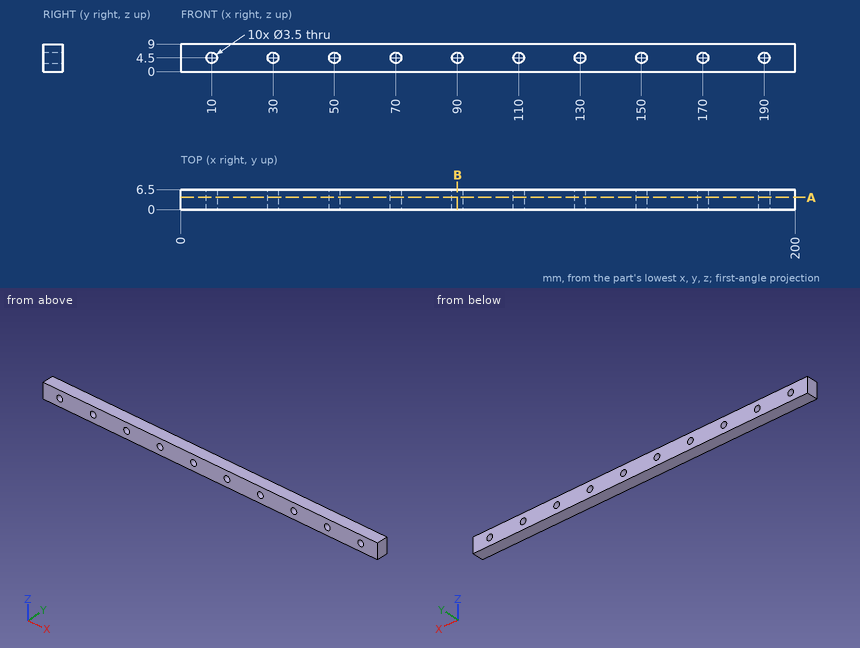
Print and shaded views of the part. All mm, measured from the part's lowest x, y and z. Round coordinates to 2 decimals unless told otherwise and drop trailing zeros. Write each loop counter-clockwise with the first axis right and the second up, starting at its lowest first coordinate (ties: lowest second). Pieces come first, ordered by that corner, then holes. Notation, with made-up numbers: (12, 20.25) -> (50, 20.25) arc R14 cw to (50, 28.25) -> close; hole circle Ø10 at (-9.75, -38.5). An arc over 180 degrees is marked (long way). Answer in a Markdown table with one row per item. Add a question column.
Item 1: Saw through at A-A, the plane y = 4. Count the separate pieces of the cut face and the enclosed holes in it, then the cut area to 3 significant figures.
Item 2: Saw through at B-B, the plane x = 90. Write the cut outline in (y, z), then the cut area to 4 significant figures.
Item 3: Drill centre line: line 1 (Z direction, x = 30, y = 1.5). Where is it in solid material? Low to high. Write a range as from..to.
Findings below:
| question | item | result |
|---|---|---|
| 1 | separate pieces | 1 |
| 1 | enclosed holes | 10 |
| 1 | area | 1,700 mm^2 |
| 2 | outline | (0, 0) -> (6.5, 0) -> (6.5, 2.75) -> (0, 2.75) -> close; (0, 6.25) -> (6.5, 6.25) -> (6.5, 9) -> (0, 9) -> close |
| 2 | area | 35.75 mm^2 |
| 3 | line 1 | z = 0..2.75, 6.25..9 |
